from build123d import *

# Parameters (mm, degrees)
SKETCH_2_R             = 1.5
SKETCH_2_R_2           = 9.5
EXTRUDE_1_DEPTH        = 4
CUT_EXTRUDE_1_DEPTH    = 124.429075185
EXTRUDE_2_DEPTH        = 4
SKETCH_7_R             = 1.5
CUT_EXTRUDE_2_DEPTH    = 155.008884812
FILLET_1_R             = 3
SKETCH_6_4_OUTSIDE_W   = 131.04
SKETCH_6_4_OUTSIDE_H   = 122.515
SKETCH_6_4_OUTSIDE_R   = 21
SKETCH_6_4_OUTSIDE_W_2 = 42
SKETCH_6_4_OUTSIDE_H_2 = 60
CUT_EXTRUDE_4_DEPTH    = 154.441846019
EXTRUDE_3_DEPTH        = 4
CUT_EXTRUDE_5_DEPTH    = 159.650559407
FILLET_2_R             = 3


with BuildPart() as part:
    # 草图2 → 凸台-拉伸1 (new body)
    with BuildSketch(Plane(origin=(0, 0, 0), x_dir=(1, 0, 0), z_dir=(0, 1, 0))):
        Polygon((0, 0), (0, 60), (40, 93.908128514), (80, 60), (80, 0), (68, 0), (68, 42), (40, 54), (12, 42), (12, 0), align=None)
        with Locations(Location((6, 32, 0), (0, 0, 270))):
            Circle(SKETCH_2_R, mode=Mode.SUBTRACT)
        with Locations(Location((6, 8, 0), (0, 0, 270))):
            Circle(SKETCH_2_R, mode=Mode.SUBTRACT)
        with Locations(Location((40, 69, 0), (0, 0, 270))):
            Circle(SKETCH_2_R_2, mode=Mode.SUBTRACT)
        with Locations(Location((74, 8, 0), (0, 0, 90))):
            Circle(SKETCH_2_R, mode=Mode.SUBTRACT)
        with Locations(Location((74, 32, 0), (0, 0, 90))):
            Circle(SKETCH_2_R, mode=Mode.SUBTRACT)
    extrude(amount=EXTRUDE_1_DEPTH)

    # 草图4 → 切除-拉伸1 (cut, through all)
    with BuildSketch(Plane(origin=(0, 4, 0), x_dir=(1, 0, 0), z_dir=(0, 1, 0))):
        with BuildLine():
            Line((24.36723091, 80.656179931), (0, 60))
            Line((0, 60), (0, 0))
            Line((0, 0), (12, 0))
            Line((12, 0), (12, 42))
            Line((12, 42), (32.756034747, 50.895443463))
            ThreePointArc((32.756034747, 50.895443463), (21.23136653, 63.709593809), (24.36723091, 80.656179931))
        make_face()
    extrude(amount=-CUT_EXTRUDE_1_DEPTH, mode=Mode.SUBTRACT)

    # 草图6 → 凸台-拉伸2 (add)
    with BuildSketch(Plane(origin=(0, 4, 0), x_dir=(1, 0, 0), z_dir=(0, 1, 0))):
        with BuildLine():
            Line((82.026334039, 60), (80, 60))
            Line((80, 60), (80, 0))
            Line((80, 0), (122, 0))
            Line((122, 0), (122, 60))
            Line((122, 60), (119.973665961, 60))
            ThreePointArc((119.973665961, 60), (101, 48), (82.026334039, 60))
        make_face()
    extrude(amount=-EXTRUDE_2_DEPTH)

    # 草图7 → 切除-拉伸2 (cut, through all)
    with BuildSketch(Plane(origin=(0, 4, 0), x_dir=(1, 0, 0), z_dir=(0, 1, 0))):
        with Locations(Location((91, 32, 0), (0, 0, 270))):
            Circle(SKETCH_7_R)
        with Locations(Location((74, 32, 0), (0, 0, 90))):
            Circle(SKETCH_7_R)
        with Locations(Location((74, 8, 0), (0, 0, 90))):
            Circle(SKETCH_7_R)
        with Locations(Location((111, 32, 0), (0, 0, 270))):
            Circle(SKETCH_7_R)
        with Locations(Location((111, 8, 0), (0, 0, 270))):
            Circle(SKETCH_7_R)
        with Locations(Location((91, 8, 0), (0, 0, 270))):
            Circle(SKETCH_7_R)
    extrude(amount=-CUT_EXTRUDE_2_DEPTH, mode=Mode.SUBTRACT)

    # 圆角1
    fillet_1_edges = [part.edges().sort_by_distance(p)[0] for p in [
        (40, 2, -93.908128514),
        (80, 2, -60),
        (68, 2, 0),
        (68, 2, -42),
        (40, 2, -54),
        (24.36723091, 2, -80.656179931),
        (32.756034747, 2, -50.895443463),
        (122, 2, 0),
    ]]
    fillet(fillet_1_edges, radius=FILLET_1_R)

    # 草图6<4> outside → 切除-拉伸4 (cut, through all)
    with BuildSketch(Plane(origin=(0, 4, 0), x_dir=(1, 0, 0), z_dir=(0, 1, 0))):
        with Locations((71.25, 46.4875)):
            Rectangle(SKETCH_6_4_OUTSIDE_W, SKETCH_6_4_OUTSIDE_H)
        with Locations((101, 69)):
            Circle(SKETCH_6_4_OUTSIDE_R, mode=Mode.SUBTRACT)
        with Locations((101, 30)):
            Rectangle(SKETCH_6_4_OUTSIDE_W_2, SKETCH_6_4_OUTSIDE_H_2, mode=Mode.SUBTRACT)
    extrude(amount=-CUT_EXTRUDE_4_DEPTH, mode=Mode.SUBTRACT)

    # 草图8 → 凸台-拉伸3 (add)
    with BuildSketch(Plane(origin=(0, 4, 0), x_dir=(1, 0, 0), z_dir=(0, 1, 0))):
        with BuildLine():
            ThreePointArc((119.973665961, 60), (101, 48), (82.026334039, 60))
            Line((82.026334039, 60), (80, 60))
            Line((80, 60), (80, 53.670290283))
            ThreePointArc((80, 53.670290283), (101, 43), (122, 53.670290283))
            Line((122, 53.670290283), (122, 60))
            Line((122, 60), (119.973665961, 60))
        make_face()
        with BuildLine():
            Line((80, 60), (82.026334039, 60))
            ThreePointArc((82.026334039, 60), (96.387353535, 89.487154331), (122, 69))
            ThreePointArc((122, 69), (121.487154331, 64.387353535), (119.973665961, 60))
            Line((119.973665961, 60), (122, 60))
            Line((122, 60), (122, 53.670290283))
            ThreePointArc((122, 53.670290283), (125.718414189, 60.937742252), (127, 69))
            ThreePointArc((127, 69), (92.937742252, 93.718414189), (80, 53.670290283))
            Line((80, 53.670290283), (80, 60))
        make_face()
    extrude(amount=-EXTRUDE_3_DEPTH)

    # 草图9 → 切除-拉伸5 (cut, through all)
    with BuildSketch(Plane.XZ):
        Polygon((110, 0), (80, -30), (80, 0), align=None)
    extrude(amount=-CUT_EXTRUDE_5_DEPTH, mode=Mode.SUBTRACT)

    # 圆角2
    fillet_2_edges = [part.edges().sort_by_distance(p)[0] for p in [
        (110, 2, 0),
        (80, 2, -30),
    ]]
    fillet(fillet_2_edges, radius=FILLET_2_R)


solid = part.part
Check sheet for the modelled part. Datum: model origin and axes. Units: mm. A direction names the side the tool comes from. Give positions to 0.01 mm unless a question says otherwise; leave off trailing zeros. Write each loop counter-clockwise with the first axis right and the second up, starting at its lowest first coordinate (ties: lowest second). Pieces come first, ordered by that corner, then holes. Notation, with made-up numbers: (14.5, 45) -> (21.5, 45) arc R13 ccw to (21.5, 67) -> close; hole circle Ø4 at (72, -35.5). An arc over 180 degrees is marked (long way). Use one line per item in the form item = value. Start each with the question number.
1. Section check A-A (y = 2). Record the cut outline in (x, z).
2. Go/stop test with flat-tipped pins: P1, Ø3.5, axis at x = 111, z = -8, coming from the +Y side; P2, Ø1, axis at x = 80.5, y = 3, coming from the +Z side; P3, Ø2, axis at y = 3, z = -40, coming from the -X side; P4, Ø1.2, axis at y = 3, z = -34.5, coming from the +X side. Record where each tip stops, or that it passes through.
3. Access from +Z, -Z, +X, -X, +Y, -Y to the whole of each face (thin tool, end or side, straight path). Record for faces 4 (the flat face through (80, 2, -42)), 5 (the flat face through (106, 0, -48)).
4. Section check C-C (z = -8). Record the cut outline in (x, y), and give its area (3 significant figures).
5. Section check B-B (x = 101). Record the cut outline in (y, z).
6. Section check D-D (x = 91). Record the cut outline in (y, z).
7. Thickness scan on line 1 along Z through (x, y) = (91, 2.6); line 2 along X through (y, z) = (1.75, -32); line 3 along Z through (x, y) = (111, 1.5). Record the ranges inside material, lowest first. Write a range as from..to.
8. Mould release check, pull along X, two halves, no side actions. Record for faces 1 (the cylindrical face through (112.487, 2.028, -32.195)), 2 (the cylindrical face through (80.235, 2.028, -30.079)), 3 (the flat face through (122, 2, -28)): pulls with the +X half, pulls with the -X half, needs draft (parallel to the pull), parting line crosses it, or undercut.
Conclusion:
q1.outline = (80, -53.67) arc R26 ccw (long way) to (122, -53.67) -> (122, -3) arc R3 ccw to (119, 0) -> (111.24, 0) arc R3 ccw to (109.12, -0.88) -> (80.88, -29.12) arc R3 ccw to (80, -31.24) -> close; hole circle Ø42 at (101, -69); hole circle Ø3 at (91, -32); hole circle Ø3 at (111, -32); hole circle Ø3 at (111, -8)
q2.P1 = 4
q2.P2 = -29
q2.P3 = 80
q2.P4 = 122
q3.face_4 = +Z, -X, +Y, -Y
q3.face_5 = +Z, -Z, +X, -X, -Y
q4.outline = (102, 0) -> (109.5, 0) -> (109.5, 4) -> (102, 4) -> close; (112.5, 0) -> (122, 0) -> (122, 4) -> (112.5, 4) -> close
q4.area = 68.0 mm²
q5.outline = (0, -95) -> (4, -95) -> (4, -90) -> (0, -90) -> close; (0, -48) -> (4, -48) -> (4, -9) -> (0, -9) -> close
q6.outline = (0, -93) -> (4, -93) -> (4, -87.47) -> (0, -87.47) -> close; (0, -50.53) -> (4, -50.53) -> (4, -33.5) -> (0, -33.5) -> close; (0, -30.5) -> (4, -30.5) -> (4, -19) -> (0, -19) -> close
q7.line_1 = -93..-87.47, -50.53..-33.5, -30.5..-19
q7.line_2 = 80..89.5, 92.5..109.5, 112.5..122
q7.line_3 = -93..-87.47, -50.53..-33.5, -30.5..-9.5, -6.5..-0.01
q8.face_1 = undercut
q8.face_2 = pulls with the -X half
q8.face_3 = pulls with the +X half
